Can you work these out from the drawing? Everything is in mm from the part's minimum corner. Give positions to 0.01 mm unless a question says otherwise; leave off trailing zeros. Order: outer loops, then holes, each group sorted by start corner. A loop starts at its lowest first (then second) coordinate and runs counter-clockwise, first axis right, second up. Notation, with made-up numbers: (10, 54) - (44, 54) arc R31 ccw to (44, 82) - close; hole circle Ø2 at (59.5, 53.5). An arc over 180 degrees is marked (long way). Answer as a JSON object with one key per item and string values.
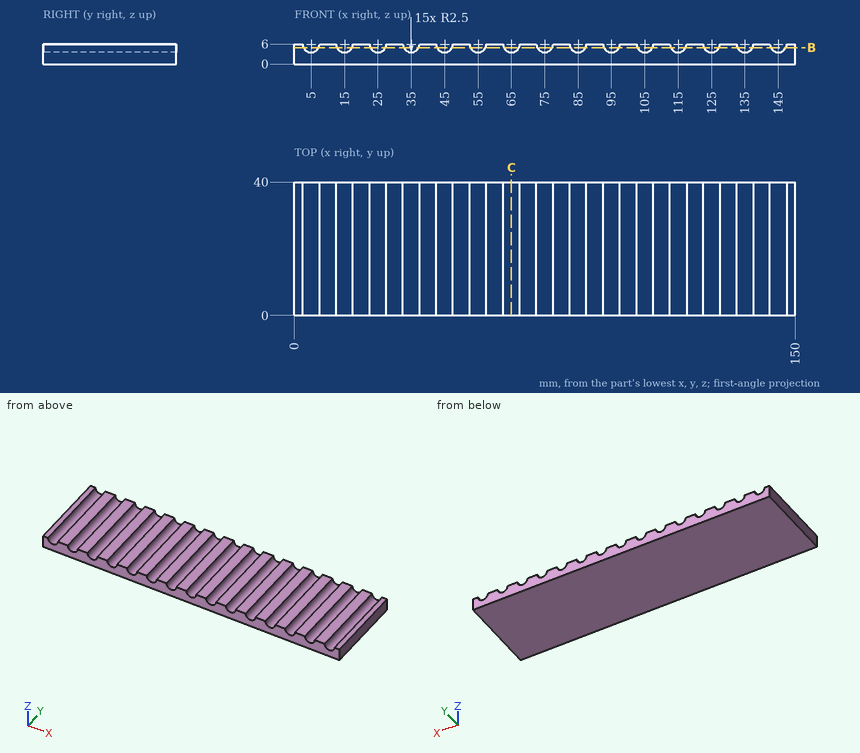
Q1. I need wall thicknesses on L1, parallel to Z at x = 103, y = 4.5. Which ranges of the line are inside material? Lowest first, please.
Recorded:
{"L1": "z = 0 to 4.5"}
Q2. I'm going to push a flat-ended pin straight in: pin 1 Ø1 at (x, y) = (115, 18) entering from +Z. Where does the tip first touch, or does it pass through?
Recorded:
{"pin 1": "stops at z = 3.55"}
Q3. If we section it at B-B, the plane z = 4.9: Count the separate pieces of the cut face and the enclosed holes in it, then the cut area to 3 significant figures.
Recorded:
{"separate pieces": "16", "enclosed holes": "0", "area": "3,310 mm^2"}
Q4. If we section it at C-C, the plane x = 65: Please give me the cut outline in (y, z), then the cut area to 3 significant figures.
Recorded:
{"outline": "(0, 0) - (40, 0) - (40, 3.5) - (0, 3.5) - close", "area": "140 mm^2"}
